The model under review builds one solid part; all positions refer to its coordinate system, in mm. A direction names the side the tool comes from. Coordinates: 2 decimals unless noted, no trailing zeros. Write each loop counter-clockwise with the first axis right and the second up, starting at its lowest first coordinate (ties: lowest second). Pieces come first, ordered by that corner, then holes. Notation, with made-up numbers: (-27.75, 77) - (5.25, 77) arc R22 ccw to (5.25, 114) - close; hole circle Ø6 at (57.25, -31). An arc over 180 degrees is marked (long way). Use one line per item in the form item = value. Start each with the question number.
```python
from build123d import *

# Parameters (mm, degrees)
SKETCH1_W               = 150
SKETCH1_H               = 150
BOSS_EXTRUDE1_DEPTH     = 5.8
CUT_EXTRUDE1_DEPTH      = 107.224479288
CUT_EXTRUDE1_DEPTH_BACK = 107.224479288
SKETCH2_R               = 1.25
SKETCH2_R_2             = 5
FILLET1_R               = 20
SKETCH3_R               = 6.25
CUT_EXTRUDE2_DEPTH      = 3.5


with BuildPart() as part:
    # Sketch1 → Boss-Extrude1 (new body)
    with BuildSketch(Plane(origin=(0, 0, 0), x_dir=(1, 0, 0), z_dir=(0, 1, 0))):
        Rectangle(SKETCH1_W, SKETCH1_H)
    extrude(amount=BOSS_EXTRUDE1_DEPTH)

    # Sketch2 → Cut-Extrude1 (cut, two sides: drawn at the far end of the back side and taken through both)
    with BuildSketch(Plane(origin=(0, 5.8, 0), x_dir=(1, 0, 0), z_dir=(0, 1, 0)).offset(-CUT_EXTRUDE1_DEPTH_BACK)):
        with Locations(Location((-61.985746634, -15.05, 0), (0, 0, 270))):
            Circle(SKETCH2_R)
        with Locations(Location((-61.985746634, 15.05, 0), (0, 0, 270))):
            Circle(SKETCH2_R)
        with Locations(Location((-21.585746634, 8.55, 0), (0, 0, 270))):
            Circle(SKETCH2_R)
        with Locations(Location((-21.585746634, -8.55, 0), (0, 0, 270))):
            Circle(SKETCH2_R)
        with Locations(Location((-57.485746634, 0, 0), (0, 0, 270))):
            Circle(SKETCH2_R_2)
    extrude(amount=CUT_EXTRUDE1_DEPTH + CUT_EXTRUDE1_DEPTH_BACK, mode=Mode.SUBTRACT)

    # Fillet1
    fillet1_edges = [part.edges().sort_by_distance(p)[0] for p in [
        (-75, 2.9, -75),
        (75, 2.9, -75),
        (75, 2.9, 75),
        (-75, 2.9, 75),
    ]]
    fillet(fillet1_edges, radius=FILLET1_R)

    # Sketch3 → Cut-Extrude2 (cut)
    with BuildSketch(Plane.XZ):
        with Locations(Location((-21.585746634, -8.55, 0), (0, 0, 270))):
            Circle(SKETCH3_R)
        with Locations(Location((-21.585746634, 8.55, 0), (0, 0, 270))):
            Circle(SKETCH3_R)
        with Locations(Location((-61.985746634, -15.05, 0), (0, 0, 270))):
            Circle(SKETCH3_R)
        with Locations(Location((-61.985746634, 15.05, 0), (0, 0, 270))):
            Circle(SKETCH3_R)
    extrude(amount=-CUT_EXTRUDE2_DEPTH, mode=Mode.SUBTRACT)


solid = part.part
```
1. The part is to be moulded in two halves that separate along X. For faces 3 (the cylindrical face through (-55.79, 1.73, -14.24)), 4 (the flat face through (75, 3, 1)), 5 (the cylindrical face through (-69.297, 2.941, 68.986)), say which applies: released by +X, released by -X, zero draft, split by the parting line, or undercut.
2. For P1, Ø11, axis at x = -61.99, z = -15.05, coming from the -Y side; P2, Ø2, axis at x = -21.59, z = -8.55, coming from the +Y side; P3, Ø2, axis at x = 59, y = 2, coming from the +Z side, all flat-tipped, find the tip position at first contact; note any pin that passes through.
3. Take a section at A-A (z = 0). State the section outline as (x, y) points, plus the area to 3 significant figures.
4. Take a section at B-B (y = 1.55). State the section outline as (x, z) points.
5. For L1, parallel to Z at x = -61, y = 3.2; L2, parallel to X at y = 3.1, z = 0; L3, parallel to X at y = 2, z = 8.55, list the stretches that pass through material, from the lowest coordinate up.
6. For faces 1 (the flat face through (-75, 3, 1)), 2 (the flat face through (-60.5, 3.5, -15)), list the 3-axis set-ups (+Z, -Z, +X, -X, +Y, -Y) from which the entire face can be reached by the end or side of a thin tool; tool diameter is ignored.
Returned:
q1.face_3 = undercut
q1.face_4 = released by +X
q1.face_5 = released by -X
q2.P1 = 3.5
q2.P2 = through
q2.P3 = 74.77
q3.outline = (-75, 0) - (-62.49, 0) - (-62.49, 5.8) - (-75, 5.8) - close; (-52.49, 0) - (75, 0) - (75, 5.8) - (-52.49, 5.8) - close
q3.area = 812 mm²
q4.outline = (-75, -55) arc R20 ccw to (-55, -75) - (55, -75) arc R20 ccw to (75, -55) - (75, 55) arc R20 ccw to (55, 75) - (-55, 75) arc R20 ccw to (-75, 55) - close; hole circle Ø12.5 at (-61.99, -15.05); hole circle Ø12.5 at (-61.99, 15.05); hole circle Ø10 at (-57.49, 0); hole circle Ø12.5 at (-21.59, -8.55); hole circle Ø12.5 at (-21.59, 8.55)
q5.L1 = -74.08 to -21.22, -8.88 to -3.56, 3.56 to 8.88, 21.22 to 74.08
q5.L2 = -75 to -62.49, -52.49 to 75
q5.L3 = -75 to -27.84, -15.34 to 75
q6.face_1 = +Z, -Z, -X, +Y, -Y
q6.face_2 = -Y
